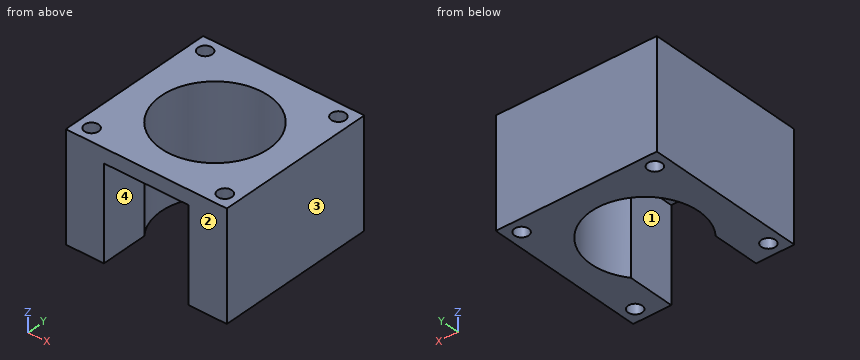
from build123d import *

# Parameters (mm, degrees)
F0_W     = 56.9976
F0_H     = 56.9976
F1_DEPTH = 38.1
F3_DEPTH = 28.4988
F4_R     = 19.05
F5_DEPTH = 38.101
F6_R     = 2.49936
F7_DEPTH = 38.101


with BuildPart() as f1:
    # F0 (on Top) → F1 (new body)
    with BuildSketch(Plane.XY):
        Rectangle(F0_W, F0_H)
    extrude(amount=F1_DEPTH)

    # F2 (on face) → F3 (cut)
    with BuildSketch(Plane.XZ.offset(28.4988)):
        Polygon((-14.9987, 0), (0, 0), (14.9987, 0), (14.9987, 32.9946), (-14.9987, 32.9946), align=None)
    extrude(amount=-F3_DEPTH, mode=Mode.SUBTRACT)

    # F4 (on face) → F5 (cut, through all)
    with BuildSketch(Plane.XY.offset(38.1)):
        Circle(F4_R)
    extrude(amount=-F5_DEPTH, mode=Mode.SUBTRACT)

    # F6 (on face) → F7 (cut, through all)
    with BuildSketch(Plane.XY.offset(38.1)):
        with Locations((-23.5712, 23.5712)):
            Circle(F6_R)
        with Locations((23.5712, 23.5712)):
            Circle(F6_R)
        with Locations((23.5712, -23.5712)):
            Circle(F6_R)
        with Locations((-23.5712, -23.5712)):
            Circle(F6_R)
    extrude(amount=-F7_DEPTH, mode=Mode.SUBTRACT)


solid = f1.part
Part model, mm, in its own coordinate system. Face numbers are marked on the shaded views. Coordinates: 2 decimals unless noted, no trailing zeros. Order: outer loops, then holes, each group sorted by start corner. A loop starts at its lowest first (then second) coordinate and runs counter-clockwise, first axis right, second up. Notation, with made-up numbers: M -7,57.5 L 49,57.5 A33 ccw 49,90.5 Z; hole C -33.75,36.25 d7. An arc over 180 degrees is marked long. Use a Markdown table: item, result.
(1) Probe L1, parallel to X at y = -12, z = 27; L2, parallel to X at y = -23, z = 3; L3, parallel to Z at x = 13, y = -19. List the from-to ranges inside material, lowest first.
A:
| item | result |
|---|---|
| L1 | x = -28.5 to -15, 15 to 28.5 |
| L2 | x = -28.5 to -26, -21.14 to -15, 15 to 21.14, 26 to 28.5 |
| L3 | z = 32.99 to 38.1 |
(2) Cut at A-A on x = 0. Write the cut outline in (y, z).
A:
| item | result |
|---|---|
| outline | M -28.5,32.99 L -19.05,32.99 L -19.05,38.1 L -28.5,38.1 Z; M 19.05,0 L 28.5,0 L 28.5,38.1 L 19.05,38.1 Z |
(3) Cut at D-D on y = -17.5. Write the cut outline in (x, z).
A:
| item | result |
|---|---|
| outline | M -28.5,0 L -15,0 L -15,32.99 L -7.53,32.99 L -7.53,38.1 L -28.5,38.1 Z; M 7.53,32.99 L 15,32.99 L 15,0 L 28.5,0 L 28.5,38.1 L 7.53,38.1 Z |
(4) Cut at C-C on z = 31. Write the cut outline in (x, y).
A:
| item | result |
|---|---|
| outline | M -28.5,-28.5 L -15,-28.5 L -15,-11.74 A19.05 cw long 15,-11.74 L 15,-28.5 L 28.5,-28.5 L 28.5,28.5 L -28.5,28.5 Z; hole C -23.57,-23.57 d5; hole C -23.57,23.57 d5; hole C 23.57,-23.57 d5; hole C 23.57,23.57 d5 |
(5) Pull direction X, two halves, no side cores. Call the marked faces 1, 2, 3 and 4: released by +X, released by -X, zero draft, split by the parting line, or undercut.
A:
| item | result |
|---|---|
| face 1 | undercut |
| face 2 | zero draft |
| face 3 | released by +X |
| face 4 | undercut |
(6) Cut at B-B on y = 0. Write the cut outline in (x, z), then the cut area to 3 significant figures.
A:
| item | result |
|---|---|
| outline | M -28.5,0 L -19.05,0 L -19.05,38.1 L -28.5,38.1 Z; M 19.05,0 L 28.5,0 L 28.5,38.1 L 19.05,38.1 Z |
| area | 720 mm^2 |
(7) Flat gauge pin, fed straight in: pin 1 (8 mm diameter, centred on x = 8, y = -16, fed in from -Z). Where does the tip first touch, or does it go through?
A:
| item | result |
|---|---|
| pin 1 | stops at z = 32.99 |
